Work out the finished part from the listing and answer in its coordinate system (mm). Round coordinates to 2 decimals unless told otherwise and drop trailing zeros. Answer in a Markdown table with one row per item.
```python
from build123d import *

# Parameters (mm, degrees)
SKETCH2_W           = 5
SKETCH2_H           = 30.99
BOSS_EXTRUDE1_DEPTH = 8.51
SKETCH3_W           = 0.635
SKETCH3_H           = 0.635
CUT_EXTRUDE1_DEPTH  = 4
CHAMFER2_SIZE       = 0.5


with BuildPart() as part:
    # Sketch2 → Boss-Extrude1 (new body)
    with BuildSketch(Plane(origin=(0, 0, 0), x_dir=(0, 0, -1), z_dir=(1, 0, 0))):
        Rectangle(SKETCH2_W, SKETCH2_H)
    extrude(amount=BOSS_EXTRUDE1_DEPTH)

    # Sketch3 → Cut-Extrude1 (cut)
    with BuildSketch(Plane.ZY):
        with Locations((-1.27, 13.965)):
            Rectangle(SKETCH3_W, SKETCH3_H)
        with Locations((1.27, 13.965)):
            Rectangle(SKETCH3_W, SKETCH3_H)
        with Locations((1.27, 11.425)):
            Rectangle(SKETCH3_W, SKETCH3_H)
        with Locations((1.27, 8.885)):
            Rectangle(SKETCH3_W, SKETCH3_H)
        with Locations((1.27, 6.345)):
            Rectangle(SKETCH3_W, SKETCH3_H)
        with Locations((1.27, 3.805)):
            Rectangle(SKETCH3_W, SKETCH3_H)
        with Locations((1.27, 1.265)):
            Rectangle(SKETCH3_W, SKETCH3_H)
        with Locations((1.27, -1.275)):
            Rectangle(SKETCH3_W, SKETCH3_H)
        with Locations((1.27, -3.815)):
            Rectangle(SKETCH3_W, SKETCH3_H)
        with Locations((1.27, -6.355)):
            Rectangle(SKETCH3_W, SKETCH3_H)
        with Locations((1.27, -8.895)):
            Rectangle(SKETCH3_W, SKETCH3_H)
        with Locations((1.27, -11.435)):
            Rectangle(SKETCH3_W, SKETCH3_H)
        with Locations((1.27, -13.975)):
            Rectangle(SKETCH3_W, SKETCH3_H)
        with Locations((-1.27, 11.425)):
            Rectangle(SKETCH3_W, SKETCH3_H)
        with Locations((-1.27, 8.885)):
            Rectangle(SKETCH3_W, SKETCH3_H)
        with Locations((-1.27, 6.345)):
            Rectangle(SKETCH3_W, SKETCH3_H)
        with Locations((-1.27, 3.805)):
            Rectangle(SKETCH3_W, SKETCH3_H)
        with Locations((-1.27, 1.265)):
            Rectangle(SKETCH3_W, SKETCH3_H)
        with Locations((-1.27, -1.275)):
            Rectangle(SKETCH3_W, SKETCH3_H)
        with Locations((-1.27, -3.815)):
            Rectangle(SKETCH3_W, SKETCH3_H)
        with Locations((-1.27, -6.355)):
            Rectangle(SKETCH3_W, SKETCH3_H)
        with Locations((-1.27, -8.895)):
            Rectangle(SKETCH3_W, SKETCH3_H)
        with Locations((-1.27, -11.435)):
            Rectangle(SKETCH3_W, SKETCH3_H)
        with Locations((-1.27, -13.975)):
            Rectangle(SKETCH3_W, SKETCH3_H)
    extrude(amount=-CUT_EXTRUDE1_DEPTH, mode=Mode.SUBTRACT)

    # Chamfer2
    chamfer2_edges = [part.edges().sort_by_distance(p)[0] for p in [
        (0, -6.6725, 1.27),
        (0, -6.355, 1.5875),
        (0, -6.0375, 1.27),
        (0, -6.355, 0.9525),
        (0, -4.1325, 1.27),
        (0, -3.815, 1.5875),
        (0, -3.4975, 1.27),
        (0, -3.815, 0.9525),
        (0, -1.5925, 1.27),
        (0, -1.275, 1.5875),
        (0, -0.9575, 1.27),
        (0, -1.275, 0.9525),
        (0, 0.9475, 1.27),
        (0, 1.265, 1.5875),
        (0, 1.5825, 1.27),
        (0, 1.265, 0.9525),
        (0, 3.4875, 1.27),
        (0, 3.805, 1.5875),
        (0, 4.1225, 1.27),
        (0, 3.805, 0.9525),
        (0, 6.0275, 1.27),
        (0, 6.345, 1.5875),
        (0, 6.6625, 1.27),
        (0, 6.345, 0.9525),
        (0, 8.5675, 1.27),
        (0, 8.885, 1.5875),
        (0, 9.2025, 1.27),
        (0, 8.885, 0.9525),
        (0, 11.1075, 1.27),
        (0, 11.425, 1.5875),
        (0, 11.7425, 1.27),
        (0, 11.425, 0.9525),
        (0, 13.6475, 1.27),
        (0, 13.965, 1.5875),
        (0, 14.2825, 1.27),
        (0, 13.965, 0.9525),
        (0, 0.9475, -1.27),
        (0, 1.265, -0.9525),
        (0, 1.5825, -1.27),
        (0, 1.265, -1.5875),
        (0, -1.5925, -1.27),
        (0, -1.275, -0.9525),
        (0, -0.9575, -1.27),
        (0, -1.275, -1.5875),
        (0, -4.1325, -1.27),
        (0, -3.815, -0.9525),
        (0, -3.4975, -1.27),
        (0, -3.815, -1.5875),
        (0, -6.6725, -1.27),
        (0, -6.355, -0.9525),
        (0, -6.0375, -1.27),
        (0, -6.355, -1.5875),
        (0, -9.2125, -1.27),
        (0, -8.895, -0.9525),
        (0, -8.5775, -1.27),
        (0, -8.895, -1.5875),
        (0, -11.7525, -1.27),
        (0, -11.435, -0.9525),
        (0, -11.1175, -1.27),
        (0, -11.435, -1.5875),
        (0, -14.2925, -1.27),
        (0, -13.975, -0.9525),
        (0, -13.6575, -1.27),
        (0, -13.975, -1.5875),
        (0, 13.965, -0.9525),
        (0, 14.2825, -1.27),
        (0, 13.965, -1.5875),
        (0, 13.6475, -1.27),
        (0, 3.4875, -1.27),
        (0, 3.805, -0.9525),
        (0, 4.1225, -1.27),
        (0, 3.805, -1.5875),
        (0, 6.0275, -1.27),
        (0, 6.345, -0.9525),
        (0, 6.6625, -1.27),
        (0, 6.345, -1.5875),
        (0, 8.5675, -1.27),
        (0, 8.885, -0.9525),
        (0, 9.2025, -1.27),
        (0, 8.885, -1.5875),
        (0, 11.1075, -1.27),
        (0, 11.425, -0.9525),
        (0, 11.7425, -1.27),
        (0, 11.425, -1.5875),
        (0, -14.2925, 1.27),
        (0, -13.975, 1.5875),
        (0, -13.6575, 1.27),
        (0, -13.975, 0.9525),
        (0, -11.7525, 1.27),
        (0, -11.435, 1.5875),
        (0, -11.1175, 1.27),
        (0, -11.435, 0.9525),
        (0, -9.2125, 1.27),
        (0, -8.895, 1.5875),
        (0, -8.5775, 1.27),
        (0, -8.895, 0.9525),
    ]]
    chamfer(chamfer2_edges, length=CHAMFER2_SIZE)


solid = part.part
```
1. Given pin 1 (0.5 mm diameter, centred on y = 4, z = 1, fed in from -X), flat-ended and moving along its own axis, determine where the tip first touches the part or whether it passes through.
Calculated:
| item | result |
|---|---|
| pin 1 | stops at x = 0.3 |
2. The part is cut by section A-A (x = 2). Count the separate pieces of the cut face and the enclosed holes in it, plus the area to 3 significant figures.
Calculated:
| item | result |
|---|---|
| separate pieces | 1 |
| enclosed holes | 24 |
| area | 145 mm² |
3. Consider line 1 along Z through (x, y) = (2.75, 1); line 2 along X through (y, z) = (-9.5, -0.8); line 3 along X through (y, z) = (4, 1.8). Determine where each line is inside the solid, lowest interval first. Write a range as from..to.
Calculated:
| item | result |
|---|---|
| line 1 | z = -2.5..-1.59, -0.95..0.95, 1.59..2.5 |
| line 2 | x = 0.21..8.51 |
| line 3 | x = 0.29..8.51 |
